The model under review builds one solid part; all positions refer to its coordinate system, in mm. A direction names the side the tool comes from. Round coordinates to 2 decimals unless told otherwise and drop trailing zeros. Write each loop counter-clockwise with the first axis right and the second up, starting at its lowest first coordinate (ties: lowest second). Pieces come first, ordered by that corner, then holes. Notation, with made-up numbers: (52, 62) -> (110, 62) arc R14 ccw to (110, 71) -> close; hole circle Ø7 at (47.25, 84). An arc over 180 degrees is marked (long way). Answer as a JSON object with one key per item and string values. Group by question number.
1) Insertion check: pin 1 Ø6 at (x, y) = (-4.5, -0.5) entering from -Z; pin 2 Ø1 at (y, z) = (0.5, 4) entering from -X; pin 3 Ø1.5 at (x, z) = (-4, 6.5) entering from +Y; pin 4 Ø7.5 at (x, y) = (-1, -0.5) entering from +Z. Each pin has a flat end and moves straight along its axis. Give the tip position at first contact, or say it passes through.
2) Machinability: for faces 4 (the cylindrical face through (-2.17, 9.76, 3.7)), 5 (the cylindrical face through (12.09, -3.81, 8.34)), 6 (the cylindrical face through (-2.17, -9.76, -2.09)), 7 (the flat face through (-0.9, 10.4, 9.2)), 8 (the flat face through (2, 5, -2.5)), which of the approach directions +Z, -Z, +X, -X, +Y, -Y give a long, thin tool a straight path to every point of the face, cutting with its end or side? Answer none if there is none.
3) We need section D-D, the plane z = 8. Write out the cut boundary in (x, y) (3 decimals), then the cut area to 3 significant figures.
4) Mouldability with a two-part tool opening along Z and no side actions: class faces 1 (the flat face through (0.9, 10.4, 0)), 2 (the flat face through (-2, 5, 10)), 3 (the cylindrical face through (-1.08, 4.88, 3.66)) as pulls with the +Z half, pulls with the -Z half, needs draft (parallel to the pull), parting line crosses it, or undercut.
5) We need section A-A, the plane x = 0. Write out the cut boundary in (y, z) (3 decimals), then the cut area to 3 significant figures.
6) To check wall thickness, follow probe 1 along Z at (x, y) = (10, -7); probe 2 along Y at (x, z) = (0, 8.75) (3 decimals); probe 3 along Y at (x, z) = (0, 2). State the ranges of each line that lie inside material, in increasing order. Write a range as [from, to].
7) We need section C-C, the plane z = 1.75. Write out the cut boundary in (x, y).
Autodesk Inventor part; units mm, degrees
ref_plane "作業平面1" through (0, 0, 3.75) normal (0, 0, 1) x (1, 0, 0)
ref_plane "YZ Plane" through (0, 0, 0) normal (1, 0, 0) x (0, 1, 0)
ref_plane "XZ Plane" through (0, 0, 0) normal (0, 1, 0) x (-1, 0, 0)
sketch "スケッチ1" plane through (0, 0, 0) normal (0, 0, 1) x (1, 0, 0)
  circle A0 centre (0, 0) radius 12.675
  circle A1 centre (0, 0) radius 5
  circle A2 centre (0, 0) radius 10
  circle A3 centre (0, 0) radius 16
  dimension "d0" = 25.35
  dimension "d1" = 10
  dimension "d2" = 20
  dimension "d3" = 32
extrude "押し出し1" add sketch "スケッチ1" along normal blind 3.75 contours A2
extrude "押し出し2" add sketch "スケッチ1" against normal blind 1.7 contours A0
extrude "押し出し3" add sketch "スケッチ1" against normal blind 2.5 contours A2
mirror "ミラー1" about plane through (0, 0, 3.75) normal (0, 0, 1) of "押し出し1", "押し出し2", "押し出し3"
ref_plane "作業平面1" through (0, 0, 3.75) normal (0, 0, 1) x (1, 0, 0)
properties part number "timing _pulley_7.5" material "アルミニウム 6061-AHC"
Here are the results:
{
 "1": {"pin 1": "stops at z = -2.5", "pin 2": "stops at x = -10", "pin 3": "stops at y = 9.46", "pin 4": "passes through"},
 "2": {"face 4": "none", "face 5": "+Z, -Z", "face 6": "-Z", "face 7": "+Z", "face 8": "-Z, +X, -X, +Y, -Y"},
 "3": {"outline": "circle Ø25.35 at (0, 0); hole circle Ø10 at (0, 0)", "area": "426 mm^2"},
 "4": {"face 1": "undercut", "face 2": "pulls with the +Z half", "face 3": "needs draft"},
 "5": {"outline": "(-12.675, -1.7) -> (-10, -1.7) -> (-10, -2.5) -> (-5, -2.5) -> (-5, 10) -> (-10, 10) -> (-10, 9.2) -> (-12.675, 9.2) -> (-12.675, 7.5) -> (-10, 7.5) -> (-10, 0) -> (-12.675, 0) -> close; (5, -2.5) -> (10, -2.5) -> (10, -1.7) -> (12.675, -1.7) -> (12.675, 0) -> (10, 0) -> (10, 7.5) -> (12.675, 7.5) -> (12.675, 9.2) -> (10, 9.2) -> (10, 10) -> (5, 10) -> close", "area": "143 mm^2"},
 "6": {"probe 1": "z = [-1.7, 0], [7.5, 9.2]", "probe 2": "y = [-12.675, -5], [5, 12.675]", "probe 3": "y = [-10, -5], [5, 10]"},
 "7": {"outline": "circle Ø20 at (0, 0); hole circle Ø10 at (0, 0)"}
}
